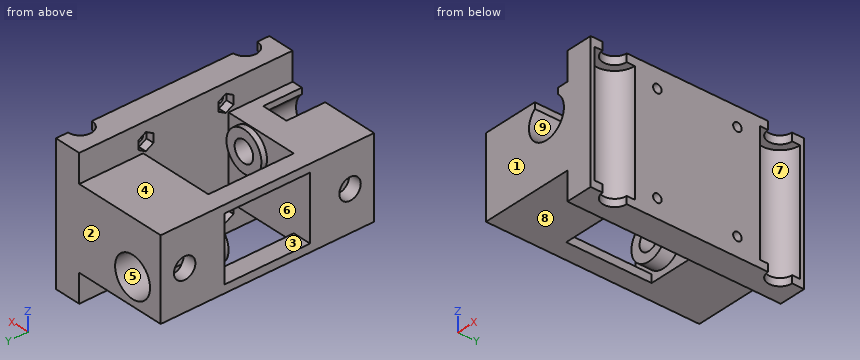
from build123d import *

# Parameters (mm, degrees)
SKETCH1_W           = 10
SKETCH1_H           = 80
BOSS_EXTRUDE1_DEPTH = 51
SKETCH2_R           = 7.525
CUT_EXTRUDE1_DEPTH  = 45.2
SKETCH3_R           = 4.5
CUT_EXTRUDE2_DEPTH  = 96.399161422
SKETCH4_W           = 30
SKETCH4_H           = 80
BOSS_EXTRUDE2_DEPTH = 35
SKETCH6_R           = 4.015
CUT_EXTRUDE3_DEPTH  = 5
SKETCH7_W           = 24
SKETCH7_H           = 32
CUT_EXTRUDE4_DEPTH  = 35
SKETCH8_W           = 28
SKETCH8_H           = 32
CUT_EXTRUDE5_DEPTH  = 101.325719534
CUT_EXTRUDE9_DEPTH  = 3
SKETCH15_R          = 1.6
CUT_EXTRUDE10_DEPTH = 103.200782776
SKETCH16_R          = 4
CUT_EXTRUDE11_DEPTH = 106.004761797
SKETCH19_R          = 4
CUT_EXTRUDE13_DEPTH = 106.004761797
BOSS_EXTRUDE3_START = 5.45
SKETCH20_R          = 7.5
SKETCH20_R_2        = 4
BOSS_EXTRUDE3_DEPTH = 5.45
BOSS_EXTRUDE4_START = 2.1
SKETCH21_R          = 7.5
SKETCH21_R_2        = 4
BOSS_EXTRUDE4_DEPTH = 2.1
BOSS_EXTRUDE5_START = -24
SKETCH22_R          = 4
BOSS_EXTRUDE5_DEPTH = 24
BOSS_EXTRUDE6_START = -24
SKETCH23_R          = 4
BOSS_EXTRUDE6_DEPTH = 24
CUT_EXTRUDE14_START = -17.8
SKETCH24_R          = 7.5
CUT_EXTRUDE14_DEPTH = 17.8
CUT_EXTRUDE15_START = -14.5
SKETCH25_R          = 7.5
CUT_EXTRUDE15_DEPTH = 14.5
CUT_EXTRUDE16_START = -14.5
CUT_EXTRUDE16_DEPTH = 14.5


with BuildPart() as part:
    # Sketch1 → Boss-Extrude1 (new body)
    with BuildSketch(Plane.XY):
        with Locations((-5, 40)):
            Rectangle(SKETCH1_W, SKETCH1_H)
    extrude(amount=BOSS_EXTRUDE1_DEPTH)

    # Sketch2 → Cut-Extrude1 (cut)
    with BuildSketch(Plane.XY.offset(48)):
        with Locations((0, 71)):
            Circle(SKETCH2_R)
        with Locations((0, 9)):
            Circle(SKETCH2_R)
    extrude(amount=-CUT_EXTRUDE1_DEPTH, mode=Mode.SUBTRACT)

    # Sketch3 → Cut-Extrude2 (cut, through all)
    with BuildSketch(Plane.XY.offset(51)):
        with Locations((0, 71)):
            Circle(SKETCH3_R)
        with Locations((0, 9)):
            Circle(SKETCH3_R)
    extrude(amount=-CUT_EXTRUDE2_DEPTH, mode=Mode.SUBTRACT)

    # Sketch4 → Boss-Extrude2 (add)
    with BuildSketch(Plane.ZY.offset(10)):
        with Locations((25.5, 40)):
            Rectangle(SKETCH4_W, SKETCH4_H)
    extrude(amount=BOSS_EXTRUDE2_DEPTH)

    # Sketch6 → Cut-Extrude3 (cut)
    with BuildSketch(Plane.ZY.offset(45)):
        with Locations((25.5, 71)):
            Circle(SKETCH6_R)
        with Locations((25.5, 9)):
            Circle(SKETCH6_R)
    extrude(amount=-CUT_EXTRUDE3_DEPTH, mode=Mode.SUBTRACT)

    # Sketch7 → Cut-Extrude4 (cut)
    with BuildSketch(Plane.ZY.offset(45)):
        with Locations((25.5, 40)):
            Rectangle(SKETCH7_W, SKETCH7_H)
    extrude(amount=-CUT_EXTRUDE4_DEPTH, mode=Mode.SUBTRACT)

    # Sketch8 → Cut-Extrude5 (cut, through all)
    with BuildSketch(Plane.XY.offset(40.5)):
        with Locations((-24, 40)):
            Rectangle(SKETCH8_W, SKETCH8_H)
    extrude(amount=-CUT_EXTRUDE5_DEPTH, mode=Mode.SUBTRACT)

    # Sketch14 → Cut-Extrude9 (cut)
    with BuildSketch(Plane.ZY.offset(10)):
        Polygon((47.262029021, 55), (45.63101451, 57.825), (42.36898549, 57.825), (40.737970979, 55), (42.36898549, 52.175), (45.63101451, 52.175), align=None)
        Polygon((10.262029021, 55), (8.63101451, 57.825), (5.36898549, 57.825), (3.737970979, 55), (5.36898549, 52.175), (8.63101451, 52.175), align=None)
        Polygon((10.262029021, 25), (8.63101451, 27.825), (5.36898549, 27.825), (3.737970979, 25), (5.36898549, 22.175), (8.63101451, 22.175), align=None)
        Polygon((47.262029021, 25), (45.63101451, 27.825), (42.36898549, 27.825), (40.737970979, 25), (42.36898549, 22.175), (45.63101451, 22.175), align=None)
    extrude(amount=-CUT_EXTRUDE9_DEPTH, mode=Mode.SUBTRACT)

    # Sketch15 → Cut-Extrude10 (cut, through all)
    with BuildSketch(Plane.ZY.offset(7)):
        with Locations((44, 55)):
            Circle(SKETCH15_R)
        with Locations((7, 55)):
            Circle(SKETCH15_R)
        with Locations((7, 25)):
            Circle(SKETCH15_R)
        with Locations((44, 25)):
            Circle(SKETCH15_R)
    extrude(amount=-CUT_EXTRUDE10_DEPTH, mode=Mode.SUBTRACT)

    # Sketch16 → Cut-Extrude11 (cut, through all)
    with BuildSketch(Plane(origin=(0, 80, 0), x_dir=(1, 0, 0), z_dir=(0, 1, 0))):
        with Locations(Location((-19, -32.664, 0), (0, 0, 270))):
            Circle(SKETCH16_R)
    extrude(amount=-CUT_EXTRUDE11_DEPTH, mode=Mode.SUBTRACT)

    # Sketch19 → Cut-Extrude13 (cut, through all)
    with BuildSketch(Plane.XZ):
        with Locations(Location((-32.925, 20.436, 0), (0, 0, 270))):
            Circle(SKETCH19_R)
    extrude(amount=-CUT_EXTRUDE13_DEPTH, mode=Mode.SUBTRACT)

    # Sketch20 → Boss-Extrude3 (add)
    with BuildSketch(Plane.XZ.offset(-56).offset(BOSS_EXTRUDE3_START)):
        with Locations(Location((-32.925, 20.436, 0), (0, 0, 90))):
            Circle(SKETCH20_R)
        with Locations(Location((-32.925, 20.436, 0), (0, 0, 270))):
            Circle(SKETCH20_R_2, mode=Mode.SUBTRACT)
    extrude(amount=-BOSS_EXTRUDE3_DEPTH)

    # Sketch21 → Boss-Extrude4 (add)
    with BuildSketch(Plane(origin=(0, 24, 0), x_dir=(1, 0, 0), z_dir=(0, 1, 0)).offset(BOSS_EXTRUDE4_START)):
        with Locations(Location((-19, -32.664, 0), (0, 0, 90))):
            Circle(SKETCH21_R)
        with Locations(Location((-19, -32.664, 0), (0, 0, 270))):
            Circle(SKETCH21_R_2, mode=Mode.SUBTRACT)
    extrude(amount=-BOSS_EXTRUDE4_DEPTH)

    # Sketch22 → Boss-Extrude5 (add)
    with BuildSketch(Plane.XZ.offset(-56).offset(BOSS_EXTRUDE5_START)):
        with Locations(Location((-19, 32.664, 0), (0, 0, 90))):
            Circle(SKETCH22_R)
    extrude(amount=BOSS_EXTRUDE5_DEPTH)

    # Sketch23 → Boss-Extrude6 (add)
    with BuildSketch(Plane(origin=(0, 24, 0), x_dir=(1, 0, 0), z_dir=(0, 1, 0)).offset(BOSS_EXTRUDE6_START)):
        with Locations(Location((-32.925, -20.436, 0), (0, 0, 90))):
            Circle(SKETCH23_R)
    extrude(amount=BOSS_EXTRUDE6_DEPTH)

    # Sketch24 → Cut-Extrude14 (cut)
    with BuildSketch(Plane(origin=(0, 80, 0), x_dir=(1, 0, 0), z_dir=(0, 1, 0)).offset(CUT_EXTRUDE14_START)):
        with Locations(Location((-32.925, -20.436, 0), (0, 0, 270))):
            Circle(SKETCH24_R)
    extrude(amount=CUT_EXTRUDE14_DEPTH, mode=Mode.SUBTRACT)

    # Sketch25 → Cut-Extrude15 (cut)
    with BuildSketch(Plane.XZ.offset(CUT_EXTRUDE15_START)):
        with Locations(Location((-19, 32.664, 0), (0, 0, 270))):
            Circle(SKETCH25_R)
    extrude(amount=CUT_EXTRUDE15_DEPTH, mode=Mode.SUBTRACT)

    # Sketch26 → Cut-Extrude16 (cut)
    with BuildSketch(Plane.XZ.offset(CUT_EXTRUDE16_START)):
        with BuildLine():
            Line((-14, 40.5), (-14, 38.254169944))
            ThreePointArc((-14, 38.254169944), (-19, 40.164), (-24, 38.254169944))
            Line((-24, 38.254169944), (-24, 40.5))
            Line((-24, 40.5), (-14, 40.5))
        make_face()
    extrude(amount=CUT_EXTRUDE16_DEPTH, mode=Mode.SUBTRACT)


solid = part.part
Check sheet for the modelled part. Datum: model origin and axes. Units: mm. Face numbers are marked on the shaded views. A direction names the side the tool comes from. Coordinates: 2 decimals unless noted, no trailing zeros. Loops run counter-clockwise (first coordinate to the right, second up) from the corner with the lowest first, then second, coordinate; pieces in that order, holes last. Notation, with made-up numbers: (-21, 60) -> (36, 60) arc R4 ccw to (36, 64) -> close; hole circle Ø2 at (8, 50.5). An arc over 180 degrees is marked (long way). Write item = value, one per line. Start each with the question number.
1. Section check B-B on z = 44. Record the cut outline in (x, y) (3 decimals).
2. Tool access check on the marked faces 5, 6, 7, 8 and 9. Record the directions out of +Z, -Z, +X, -X, +Y, -Y that give a thin tool (end or side, any length) a straight path to the whole face; none if there is none.
3. Section check D-D on y = 9. Record the cut outline in (x, z) (3 decimals).
4. Depth check by flat-ended pin: P1, Ø1.5, axis at x = -35, y = 12.5, coming from the -Z side; P2, Ø4, axis at y = 25, z = 7, coming from the -X side; P3, Ø12, axis at x = -19, z = 9.5, coming from the +Y side; P4, Ø6.5, axis at y = 9, z = 25.5, coming from the -X side. Enter the tip coordinate at first touch or a pass-through.
5. Draft check along Y on the marked faces 1, 2, 3 and 4. Enter one of: released by +Y, released by -Y, zero draft, split by the parting line, or undercut.
6. Section check C-C on x = -9. Record the cut outline in (y, z) (3 decimals), then the cut area to 3 significant figures.
7. Material ranges on line 1 (Y direction, x = -8, z = 6) (3 decimals); line 2 (Y direction, x = -43.3, z = 25.5) (3 decimals); line 3 (Y direction, x = -17.5, z = 23.5), recorded low to high.
8. Section check A-A on x = -19. Record the cut outline in (y, z), then the cut area to 3 significant figures.
Responses:
q1.outline = (-10, 0) -> (0, 0) -> (0, 1.475) arc R7.525 cw to (0, 16.525) -> (0, 23.4) -> (-7, 23.4) -> (-7, 22.175) -> (-10, 22.175) -> close; (-10, 27.825) -> (-7, 27.825) -> (-7, 26.6) -> (0, 26.6) -> (0, 53.4) -> (-7, 53.4) -> (-7, 52.175) -> (-10, 52.175) -> close; (-10, 57.825) -> (-7, 57.825) -> (-7, 56.6) -> (0, 56.6) -> (0, 63.475) arc R7.525 cw to (0, 78.525) -> (0, 80) -> (-10, 80) -> close
q2.face_5 = +Y
q2.face_6 = none
q2.face_7 = +X
q2.face_8 = -Z, -X, +Y, -Y
q2.face_9 = -Y
q3.outline = (-45, 10.5) -> (-10, 10.5) -> (-10, 0) -> (-4.5, 0) -> (-4.5, 2.8) -> (-7.525, 2.8) -> (-7.525, 48) -> (-4.5, 48) -> (-4.5, 51) -> (-10, 51) -> (-10, 40.5) -> (-14, 40.5) -> (-14, 38.254) arc R7.5 cw (long way) to (-24, 38.254) -> (-24, 40.5) -> (-45, 40.5) -> (-45, 29.515) -> (-40, 29.515) -> (-40, 21.485) -> (-45, 21.485) -> close
q4.P1 = 10.5
q4.P2 = -7
q4.P3 = 80
q4.P4 = -40
q5.face_1 = released by -Y
q5.face_2 = released by +Y
q5.face_3 = undercut
q5.face_4 = zero draft
q6.outline = (0, 0) -> (80, 0) -> (80, 51) -> (0, 51) -> close; hole (22.175, 5.369) -> (25, 3.738) -> (27.825, 5.369) -> (27.825, 8.631) -> (25, 10.262) -> (22.175, 8.631) -> close; hole (22.175, 42.369) -> (25, 40.738) -> (27.825, 42.369) -> (27.825, 45.631) -> (25, 47.262) -> (22.175, 45.631) -> close; hole (52.175, 5.369) -> (55, 3.738) -> (57.825, 5.369) -> (57.825, 8.631) -> (55, 10.262) -> (52.175, 8.631) -> close; hole (52.175, 42.369) -> (55, 40.738) -> (57.825, 42.369) -> (57.825, 45.631) -> (55, 47.262) -> (52.175, 45.631) -> close
q6.area = 3,970 mm2
q7.line_1 = 0 to 22.175, 27.825 to 52.175, 57.825 to 80
q7.line_2 = 0 to 4.985, 13.015 to 24, 56 to 66.985, 75.015 to 80
q7.line_3 = 0 to 24, 56 to 80
q8.outline = (0, 10.5) -> (24, 10.5) -> (24, 25.16) -> (26.1, 25.16) -> (26.1, 28.66) -> (14.5, 28.66) -> (14.5, 25.16) -> (0, 25.16) -> close; (14.5, 36.66) -> (26.1, 36.66) -> (26.1, 40.16) -> (24, 40.16) -> (24, 40.5) -> (14.5, 40.5) -> close; (56, 10.5) -> (80, 10.5) -> (80, 40.5) -> (56, 40.5) -> close
q8.area = 1,160 mm2
